```python
from build123d import *

# Parameters (mm, degrees)
F0_R     = 15.875
F1_DEPTH = 41
F2_W     = 7
F2_H     = 9.5
F3_DEPTH = 25
F5_D     = 11
F5_DEPTH = 32
F5_TIP   = 3.3047334047


with BuildPart() as f1:
    # F0 (on Top) → F1 (new body)
    with BuildSketch(Plane.XY):
        Circle(F0_R)
    extrude(amount=F1_DEPTH)

    # F2 (on Front) → F3 (cut, symmetric)
    with BuildSketch(Plane.XZ):
        with Locations((-13, 36.25)):
            Rectangle(F2_W, F2_H)
        with Locations((13, 36.25)):
            Rectangle(F2_W, F2_H)
    extrude(amount=F3_DEPTH, both=True, mode=Mode.SUBTRACT)

    # F5
    with Locations(Plane.XY.offset(41)):
        with Locations((0, 0)):
            Hole(F5_D / 2, depth=F5_DEPTH)
            with Locations((0, 0, -(F5_DEPTH + F5_TIP / 2))):  # 118° drill point
                Cone(0, F5_D / 2, F5_TIP, mode=Mode.SUBTRACT)


solid = f1.part
```
Could you check a few things on this model? Use its own coordinates, in mm. A direction names the side the tool comes from. Give positions to 0.01 mm unless a question says otherwise; leave off trailing zeros. Loops run counter-clockwise (first coordinate to the right, second up) from the corner with the lowest first, then second, coordinate; pieces in that order, holes last. Notation, with made-up numbers: (84, 83.5) - (92, 83.5) arc R6 cw to (92, 92.5) - close; hole circle Ø7 at (-30.75, 70). An arc over 180 degrees is marked (long way). Answer in a Markdown table with one row per item. Add a question column.
Q1. We'd pull the mould along Y, two halves only. Please class faces 1 (the face through (14.664, -6.08, 20.213)), 2 (the face through (0.91, 0.29, 6.27)), 3 (the face through (-4, 4, 41)): +Y half, -Y half, draft (parallel to the pull), parting line (faces both ways), or undercut.
Q2. Which directions (+Z, -Z, +X, -X, +Y, -Y) give clear straight access to the entire face, cutting with the end or side of a thin tool? Please do faces 4 (the face through (0, 0, 0)), 5 (the face through (1.19, -5.37, 24.78)), 6 (the face through (12, 0, 31.5)), 7 (the face through (-12, 0, 31.5)).
Q3. If we section it at B-B (y = -6): List the corners of the cut face in (x, z) for me, plus the area to 3 significant figures.
Q4. If we section it at A-A (z = 32.5): List the corners of the cut face in (x, y) for me (3 decimals).
Q5. Please list where these lines run through material, in increasing order: L1, parallel to Y at x = 0, z = 25.5 (3 decimals); L2, parallel to Z at x = 13.5, y = -2. Write a range as from..to.
Q6. If we section it at D-D (y = 10): List the corners of the cut face in (x, z) for me.
Q7. For pin 1 (2 mm diameter, centred on y = -8, z = 16.5, fed in from +X); pin 2 (10.5 mm diameter, centred on y = 5.5, z = 37, fed in from +X); pin 3 (8 mm diameter, centred on y = 12, z = 34.5, fed in from +X), each with a flat end and sliding along its axis, tell me the tip position at first contact or that it passes through.
Q8. If we section it at C-C (x = -9): List the corners of the cut face in (y, z) for me.
The answers:
| question | item | result |
|---|---|---|
| 1 | face 1 | parting line |
| 1 | face 2 | undercut |
| 1 | face 3 | draft |
| 2 | face 4 | -Z, +X, -X, +Y, -Y |
| 2 | face 5 | +Z |
| 2 | face 6 | +Z, +X, +Y, -Y |
| 2 | face 7 | +Z, -X, +Y, -Y |
| 3 | outline | (-14.7, 0) - (14.7, 0) - (14.7, 31.5) - (9.5, 31.5) - (9.5, 41) - (-9.5, 41) - (-9.5, 31.5) - (-14.7, 31.5) - close |
| 3 | area | 1,110 mm^2 |
| 4 | outline | (-9.5, -12.719) arc R15.875 ccw to (9.5, -12.719) - (9.5, 12.719) arc R15.875 ccw to (-9.5, 12.719) - close; hole circle Ø11 at (0, 0) |
| 5 | L1 | y = -15.875..-5.5, 5.5..15.875 |
| 5 | L2 | z = 0..31.5 |
| 6 | outline | (-12.33, 0) - (12.33, 0) - (12.33, 31.5) - (9.5, 31.5) - (9.5, 41) - (-9.5, 41) - (-9.5, 31.5) - (-12.33, 31.5) - close |
| 7 | pin 1 | stops at x = 14.25 |
| 7 | pin 2 | stops at x = 9.5 |
| 7 | pin 3 | stops at x = 12.83 |
| 8 | outline | (-13.08, 0) - (13.08, 0) - (13.08, 41) - (-13.08, 41) - close |
